Build history of the part. All positions in model axes, mm. Give positions to 0.01 mm unless a question says otherwise; leave off trailing zeros. Write each loop counter-clockwise with the first axis right and the second up, starting at its lowest first coordinate (ties: lowest second). Pieces come first, ordered by that corner, then holes. Notation, with made-up numbers: M 31.5,-35.5 L 50.5,-35.5 A18 ccw 50.5,-30.5 Z; hole C 37.25,79.5 d2. An arc over 180 degrees is marked long. Return JSON: item names as keys, results as strings. Group by question number.
Q1. Band-saw the part on A-A, the plane z = 0. Give the cut face in (x, y).
Q2. Band-saw the part on D-D, the plane z = 14. Give the cut face in (x, y), then the cut area to 3 significant figures.
Q3. Band-saw the part on C-C, the plane x = 10.5. Give the cut face in (y, z).
Q4. Wall check: probe 1 along Y at (x, z) = (12.5, 0); probe 2 along Z at (x, y) = (7, 54); probe 3 along Z at (x, y) = (14.5, 32.5). Give the ranges that are in metal, low to high.
Q5. Band-saw the part on B-B, the plane y = 37. Give the cut face in (x, z).
Q6. Flat gauge pins, fed straight in: pin 1 Ø1.5 at (x, y) = (19.5, 40) entering from +Z; pin 2 Ø1.5 at (x, y) = (-20.5, 15.5) entering from +Z; pin 3 Ø2 at (x, y) = (0, 54) entering from -Z. Where does each tip first touch, or does it go through?
from build123d import *

# Parameters (mm, degrees)
BOSS_EXTRUDE1_DEPTH     = 76.2
CUT_EXTRUDE1_REACH      = 104.716
CUT_EXTRUDE1_END_RADIUS = 88.9
SKETCH2_R               = 25.4


with BuildPart() as part:
    # Sketch1 → Boss-Extrude1 (new body)
    with BuildSketch(Plane(origin=(0, 0, 0), x_dir=(1, 0, 0), z_dir=(0, 1, 0))):
        with BuildLine():
            Line((0, 63.5), (0, -63.5))
            ThreePointArc((0, -63.5), (26.682960533, 0), (0, 63.5))
        make_face()
    extrude(amount=BOSS_EXTRUDE1_DEPTH)

    # Cut-Extrude1: up to this cylinder (the profile starts inside it)
    cut_extrude1_end = Plane(origin=(-62.217039467, 40.64, 0), z_dir=(0, -1, 0)) * Cylinder(CUT_EXTRUDE1_END_RADIUS, 388.232, mode=Mode.PRIVATE)
    # Sketch2 → Cut-Extrude1 (cut, up to the surface)
    with BuildSketch(Plane.ZY, mode=Mode.PRIVATE) as cut_extrude1_sk1:
        with Locations((0, 40.64)):
            Circle(SKETCH2_R)
    cut_extrude1_tool1 = extrude(cut_extrude1_sk1.sketch, amount=-CUT_EXTRUDE1_REACH, mode=Mode.PRIVATE) & cut_extrude1_end
    add(cut_extrude1_tool1.solids().sort_by_distance((0, 40.64, 0))[0], mode=Mode.SUBTRACT)

    # Mirror1: part across plane


with BuildPart() as part_1:
    add(part.part)
    add(part.part.mirror(Plane(origin=(0, 76.2, -63.5), x_dir=(0, 0, 1), z_dir=(1, 0, 0))))


solid = part_1.part
From the geometry:
{
 "1": {"outline": "M -26.68,0 L 26.68,0 L 26.68,15.24 L -26.68,15.24 Z; M -26.68,66.04 L 26.68,66.04 L 26.68,76.2 L -26.68,76.2 Z"},
 "2": {"outline": "M -25.57,0 L 25.57,0 L 25.57,19.45 L -25.57,19.45 Z; M -25.57,61.83 L 25.57,61.83 L 25.57,76.2 L -25.57,76.2 Z", "area": "1,730 mm^2"},
 "3": {"outline": "M 0,-51.14 L 76.2,-51.14 L 76.2,51.14 L 0,51.14 Z; hole C 40.64,0 d50.8"},
 "4": {"probe 1": "y = 0 to 15.24, 66.04 to 76.2", "probe 2": "z = -55.79 to -21.6, 21.6 to 55.79", "probe 3": "z = -44.92 to -24.06, 24.06 to 44.92"},
 "5": {"outline": "M -23.05,-25.14 A88.9 ccw 0,-63.5 A88.9 ccw 23.05,-25.14 Z; M -23.05,25.14 L 23.05,25.14 A88.9 ccw 0,63.5 A88.9 ccw Z"},
 "6": {"pin 1": "stops at z = 36.71", "pin 2": "stops at z = 34.42", "pin 3": "stops at z = -63.5"}
}
